Part model, mm, in its own coordinate system. A direction names the side the tool comes from. Round coordinates to 2 decimals unless told otherwise and drop trailing zeros. Write each loop counter-clockwise with the first axis right and the second up, starting at its lowest first coordinate (ties: lowest second). Pieces come first, ordered by that corner, then holes.
1) Saw through at A-A on y = 49.5. Write the cut outline in (x, z) (3 decimals).
2) Flat gauge pins, fed straight in: pin 1 (1 mm diameter, centred on x = 58, y = 10, fed in from +Z); pin 2 (14 mm diameter, centred on y = 16.5, z = 18, fed in from -X) (3 decimals); pin 3 (22 mm diameter, centred on x = 41.5, z = 36.5, fed in from +Y). Where does each tip first touch, or does it go through?
3) Which spindle directions (+Z, -Z, +X, -X, +Y, -Y) get a long thin tool onto all of the face, cutting with end or side? Do faces 4 (the cylindrical face through (45.8, -0.4, 38.1)), 5 (the flat face through (-4, -3.175, 36)), 6 (the flat face through (22.225, 14, 18)). Say none if no direction does.
4) Pull direction X, two halves, no side cores. Call faces 1 (the flat face through (60.325, 0, 40)), 2 (the flat face through (60.325, 0, 64)), 3 (the flat face through (86, 0, 38.1)): +X half, -X half, draft (parallel to the pull), parting line (faces both ways), or undercut.
5) Drill centre lines: L1, parallel to X at y = -17, z = 21 (3 decimals); L2, parallel to X at y = -8.5, z = 9 (3 decimals); L3, parallel to X at y = -12, z = 38.5 (3 decimals). Where is each one in solid material? Low to high.
```python
from build123d import *

# Parameters (mm, degrees)
F1_DEPTH = 63.5
F0_W     = 25.4
F0_H     = 4.7752
F0_H_2   = 19.05
F0_H_3   = 4.7498
F2_DEPTH = 25.4
F4_DEPTH = 3.175
F5_R     = 12.7


with BuildPart() as f1:
    # F0 (on Front) → F1 (new body, symmetric)
    with BuildSketch(Plane.XZ):
        Polygon((41.275, -9.525), (41.275, 9.525), (22.225, 9.525), (-41.275, 9.525), (-41.275, -9.525), align=None)
    extrude(amount=F1_DEPTH, both=True)

    # F0 (on Front) → F2 (join, symmetric)
    with BuildSketch(Plane.XZ):
        with BuildLine():
            Line((22.225, 9.525), (41.275, 9.525))
            Line((41.275, 9.525), (41.275, 27.0002))
            ThreePointArc((41.275, 27.0002), (45.9246798487, 38.2255201513), (57.15, 42.8752))
            Line((57.15, 42.8752), (60.325, 42.8752))
            Line((60.325, 42.8752), (60.325, 61.9252))
            Line((60.325, 61.9252), (57.15, 61.9252))
            ThreePointArc((57.15, 61.9252), (32.4542956671, 51.6959043329), (22.225, 27.0002))
            Line((22.225, 27.0002), (22.225, 9.525))
        make_face()
        with Locations((73.025, 40.4876)):
            Rectangle(F0_W, F0_H)
        with Locations((73.025, 52.4002)):
            Rectangle(F0_W, F0_H_2)
        with Locations((73.025, 64.3001)):
            Rectangle(F0_W, F0_H_3)
    extrude(amount=F2_DEPTH, both=True)

    # F0 (on Front) → F3 (revolve)
    with BuildSketch(Plane.XZ):
        Polygon((85.725, 61.9252), (85.725, 42.8752), (85.725, 38.1), (111.125, 38.1), (111.125, 66.675), (85.725, 66.675), align=None)
    revolve(axis=Axis((85.725, 0, 52.3875), (0, 0, 1)))

    # F0 (on Front) → F4 (join, symmetric)
    with BuildSketch(Plane.XZ):
        with BuildLine():
            Line((-41.275, 9.525), (22.225, 9.525))
            Line((22.225, 9.525), (22.225, 27.0002))
            ThreePointArc((22.225, 27.0002), (32.4542956671, 51.6959043329), (57.15, 61.9252))
            add(Edge.make_bspline(
                [(-41.275, 9.525), (-40.8581793308, 53.2651096582), (7.8326556832, 62.0646551251), (57.15, 61.9252)],
                knots=[0, 0, 0, 0, 111.5045361635, 111.5045361635, 111.5045361635, 111.5045361635], degree=3))
        make_face()
    extrude(amount=F4_DEPTH, both=True)

    # F5
    f5_edges = [f1.edges().sort_by_distance(p)[0] for p in [
        (85.725, 25.4, 52.3875),
        (73.025, 25.4, 66.675),
        (73.025, -25.4, 66.675),
        (111.125, 0, 66.675),
    ]]
    fillet(f5_edges, radius=F5_R)


solid = f1.part
```
Completed:
1. outline: (-41.275, -9.525) - (41.275, -9.525) - (41.275, 9.525) - (-41.275, 9.525) - close
2. pin 1: stops at z = 61.93
2. pin 2: stops at x = 22.225
2. pin 3: stops at y = 25.4
3. face 4: -Z, +Y, -Y
3. face 5: +Z, -X, -Y
3. face 6: +Z, -X, +Y
4. face 1: undercut
4. face 2: -X half
4. face 3: draft
5. L1: x = 22.225 to 41.275
5. L2: x = -41.275 to 41.275
5. L3: x = 24.173 to 46.206, 60.325 to 108.112
